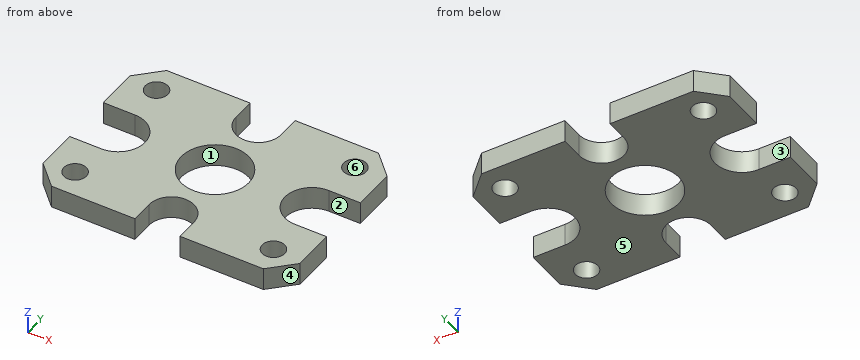
from build123d import *

# Parameters (mm, degrees)
SKETCH1_R           = 5
SKETCH1_R_2         = 15
BOSS_EXTRUDE1_DEPTH = 5


with BuildPart() as part:
    # Sketch1 → Boss-Extrude1 (new, symmetric)
    with BuildSketch(Plane.XY):
        with BuildLine():
            Line((-57, -31), (-47, -41))
            Line((-47, -41), (-10, -41))
            Line((-10, -41), (-10, -31))
            ThreePointArc((-10, -31), (0, -21), (10, -31))
            Line((10, -31), (10, -41))
            Line((10, -41), (47, -41))
            Line((47, -41), (57, -31))
            Line((57, -31), (57, -12))
            Line((57, -12), (43, -12))
            ThreePointArc((43, -12), (31, 0), (43, 12))
            Line((43, 12), (57, 12))
            Line((57, 12), (57, 31))
            Line((57, 31), (47, 41))
            Line((47, 41), (10, 41))
            Line((10, 41), (10, 31))
            ThreePointArc((10, 31), (0, 21), (-10, 31))
            Line((-10, 31), (-10, 41))
            Line((-10, 41), (-47, 41))
            Line((-47, 41), (-57, 31))
            Line((-57, 31), (-57, 12))
            Line((-57, 12), (-43, 12))
            ThreePointArc((-43, 12), (-31, 0), (-43, -12))
            Line((-43, -12), (-57, -12))
            Line((-57, -12), (-57, -31))
        make_face()
        with Locations((-44, -29)):
            Circle(SKETCH1_R, mode=Mode.SUBTRACT)
        with Locations(Location((-44, 29, 0), (0, 0, 180))):
            Circle(SKETCH1_R, mode=Mode.SUBTRACT)
        with Locations(Location((44, -29, 0), (0, 0, 180))):
            Circle(SKETCH1_R, mode=Mode.SUBTRACT)
        with Locations((44, 29)):
            Circle(SKETCH1_R, mode=Mode.SUBTRACT)
        Circle(SKETCH1_R_2, mode=Mode.SUBTRACT)
    extrude(amount=BOSS_EXTRUDE1_DEPTH, both=True)


solid = part.part
The listing builds one solid part. Answer for the finished solid, in the listing's coordinates (mm). Face numbers are marked on the shaded views. A direction names the side the tool comes from. Coordinates: 2 decimals unless noted, no trailing zeros. Order: outer loops, then holes, each group sorted by start corner. A loop starts at its lowest first (then second) coordinate and runs counter-clockwise, first axis right, second up.
Q1. A cutting plane is placed at C-C, the plane y = -10.5. Write down the section's boundary in (x, z).
Q2. Given P1, Ø9, axis at x = 44, y = 29, coming from the -Z side; P2, Ø3, axis at y = -36, z = -2, coming from the -X side; P3, Ø5, axis at y = -35, z = -1.5, coming from the +X side; P4, Ø13, axis at x = 44, y = -29, coming from the -Z side, each flat-ended and moving along its own axis, determine where each tip first touches the part or whether it passes through.
Q3. A cutting plane is placed at D-D, the plane y = -29. Write down the section's boundary in (x, z).
Q4. Which of the six approach directions +Z, -Z, +X, -X, +Y, -Y give full straight-line access (tool end or side, diameter ignored) to the marked faces 1, 2 and 3?
Q5. A cutting plane is placed at A-A, the plane x = 0. Write down the section's boundary in (y, z), and give its area (3 significant figures).
Q6. A cutting plane is placed at B-B, the plane z = 3. State how many separate pieces and enclosed holes the cut face has, and give its area (3 significant figures).
Q7. For a pull along Y with two mould halves and no side action, classify the marked faces 4, 5 and 6 as pulls with the +Y half, pulls with the -Y half, needs draft (parallel to the pull), parting line crosses it, or undercut.
Q8. Consider line 1 (Y direction, x = -44, z = 1.75); line 2 (X direction, y = 26.5, z = -3); line 3 (X direction, y = -25.5, z = 0.5). Determine where each line is inside the solid, lowest interval first.
Answers follow:
1. outline: (-37.19, -5) - (-10.71, -5) - (-10.71, 5) - (-37.19, 5) - close; (10.71, -5) - (37.19, -5) - (37.19, 5) - (10.71, 5) - close
2. P1: passes through
2. P2: stops at x = -53.5
2. P3: stops at x = 55.5
2. P4: stops at z = -5
3. outline: (-57, -5) - (-49, -5) - (-49, 5) - (-57, 5) - close; (-39, -5) - (-9.8, -5) - (-9.8, 5) - (-39, 5) - close; (9.8, -5) - (39, -5) - (39, 5) - (9.8, 5) - close; (49, -5) - (57, -5) - (57, 5) - (49, 5) - close
4. face 1: +Z, -Z
4. face 2: +Z, -Z, +X
4. face 3: +Z, -Z, -X
5. outline: (-21, -5) - (-15, -5) - (-15, 5) - (-21, 5) - close; (15, -5) - (21, -5) - (21, 5) - (15, 5) - close
5. area: 120 mm2
6. separate pieces: 1
6. enclosed holes: 5
6. area: 6,290 mm2
7. face 4: pulls with the -Y half
7. face 5: needs draft
7. face 6: undercut
8. line 1: y = -41 to -34, -24 to -12, 12 to 24, 34 to 41
8. line 2: x = -57 to -48.33, -39.67 to -8.93, 8.93 to 39.67, 48.33 to 57
8. line 3: x = -57 to -47.57, -40.43 to -8.35, 8.35 to 40.43, 47.57 to 57
